Work out the finished part from the listing and answer in its coordinate system (mm). A direction names the side the tool comes from. Round coordinates to 2 decimals unless told otherwise and drop trailing zeros. Loops run counter-clockwise (first coordinate to the right, second up) from the corner with the lowest first, then second, coordinate; pieces in that order, holes last.
```python
from build123d import *

# Parameters (mm, degrees)
SCHIZZO1_W                   = 50
SCHIZZO1_H                   = 23
ESTRUSIONE_ESTRUSIONE1_DEPTH = 100
SCHIZZO2_W                   = 10
SCHIZZO2_H                   = 50
ESTRUSIONE_ESTRUSIONE2_DEPTH = 30
M7_CLEARANCE_HOLE1_D         = 7.6
ESTRUSIONE_ESTRUSIONE3_DEPTH = 60
NERVATURA2_REACH             = 125.73
SCHIZZO10_WALL_W             = 291.885494398
SCHIZZO10_WALL_H             = 5
SCHIZZO11_W                  = 30
SCHIZZO11_H                  = 30
ESTRUSIONE_ESTRUSIONE4_DEPTH = 8
TAGLIO_ESTRUSIONE1_DEPTH     = 8
RACCORDO1_R                  = 10
SMUSSO2_SIZE                 = 2
RACCORDO2_R                  = 5
SCHIZZO17_W                  = 25
SCHIZZO17_H                  = 25
ESTRUSIONE_ESTRUSIONE8_DEPTH = 3
M7_CLEARANCE_HOLE2_D         = 7.6


with BuildPart() as part:
    # Schizzo1 → Estrusione-Estrusione1 (new body)
    with BuildSketch(Plane.YZ):
        with Locations((0, 11.5)):
            Rectangle(SCHIZZO1_W, SCHIZZO1_H)
    extrude(amount=ESTRUSIONE_ESTRUSIONE1_DEPTH)

    # Schizzo2 → Estrusione-Estrusione2 (add)
    with BuildSketch(Plane.XY.offset(23)):
        with Locations((35, 0)):
            Rectangle(SCHIZZO2_W, SCHIZZO2_H)
    extrude(amount=ESTRUSIONE_ESTRUSIONE2_DEPTH)

    # M7 Clearance Hole1 (through all)
    with Locations(Plane.ZY.offset(-30)):
        with Locations((38, 0)):
            Hole(M7_CLEARANCE_HOLE1_D / 2)

    # Schizzo5 → Estrusione-Estrusione3 (add)
    with BuildSketch(Plane.YZ.offset(40)):
        Polygon((-2.124355653, 23), (2.124355653, 23), (4, 30), (-4, 30), align=None)
    extrude(amount=ESTRUSIONE_ESTRUSIONE3_DEPTH)

    # Schizzo10 wall → Nervatura2 (add, up to next)
    with BuildSketch(Plane(origin=(55, -25, 38), x_dir=(0.707106781187, 0, -0.707106781187), z_dir=(0.707106781187, 0, 0.707106781187)), mode=Mode.PRIVATE) as nervatura2_sk1:
        with Locations((0, 2.5)):
            Rectangle(SCHIZZO10_WALL_W, SCHIZZO10_WALL_H)
    nervatura2_tool1 = extrude(nervatura2_sk1.sketch, amount=-NERVATURA2_REACH, mode=Mode.PRIVATE) - part.part
    nervatura2 = nervatura2_tool1.solids().sort_by_distance((55, -25, 38))[0]
    add(nervatura2)

    # Specchia2: Nervatura2 across plane
    add(nervatura2.mirror(Plane.ZX))

    # Schizzo11 → Estrusione-Estrusione4 (add)
    with BuildSketch(Plane.YZ.offset(40)):
        with Locations((0, 38)):
            Rectangle(SCHIZZO11_W, SCHIZZO11_H)
    extrude(amount=ESTRUSIONE_ESTRUSIONE4_DEPTH)

    # Schizzo13 → Taglio-Estrusione1 (cut)
    with BuildSketch(Plane.YZ.offset(48)):
        Polygon((-6.5, 41.75277675), (-6.5, 34.24722325), (0, 30.494446501), (6.5, 34.24722325), (6.5, 41.75277675), (6.5, 53), (-6.5, 53), align=None)
    extrude(amount=-TAGLIO_ESTRUSIONE1_DEPTH, mode=Mode.SUBTRACT)

    # Schizzo16 → CSK for M3.5 Oval Head Machine Screw1 (revolve, cut)
    with BuildSketch(Plane(origin=(15, -12.5, 23), x_dir=(0, -1, 0), z_dir=(1, 0, 0))):
        Polygon((0, 0), (0, 31.171678207), (1.95, 30), (1.95, 2.15), (4.1, 0), align=None)
    csk_for_m3_5_oval_head_machine_screw1 = revolve(axis=Axis((15, -12.5, 29.35), (0, 0, -1)), mode=Mode.SUBTRACT)

    # Specchia3: CSK for M3.5 Oval Head Machine Screw1 across plane
    add(csk_for_m3_5_oval_head_machine_screw1.mirror(Plane.ZY.offset(-50)), mode=Mode.SUBTRACT)

    # Specchia3 at the second plane: CSK for M3.5 Oval Head Machine Screw1 across plane
    add(csk_for_m3_5_oval_head_machine_screw1.mirror(Plane.ZX), mode=Mode.SUBTRACT)

    # Specchia3 at the second plane copy 1 ske → Specchia3 at the second plane copy 1 (revolve, cut)
    with BuildSketch(Plane(origin=(85, 12.5, 23), x_dir=(0, 1, 0), z_dir=(-1, 0, 0))):
        Polygon((0, 0), (0, 31.171678207), (1.95, 30), (1.95, 2.15), (4.1, 0), align=None)
    revolve(axis=Axis((85, 12.5, 29.35), (0, 0, -1)), mode=Mode.SUBTRACT)

    # Raccordo1
    raccordo1_edges = [part.edges().sort_by_distance(p)[0] for p in [
        (100, 25, 11.5),
        (100, -25, 11.5),
        (0, 25, 11.5),
        (0, -25, 11.5),
    ]]
    fillet(raccordo1_edges, radius=RACCORDO1_R)

    # Smusso2
    smusso2_edges = [part.edges().sort_by_distance(p)[0] for p in [
        (44, 6.5, 53),
        (44, -6.5, 53),
    ]]
    chamfer(smusso2_edges, length=SMUSSO2_SIZE)

    # Raccordo2
    raccordo2_edges = [part.edges().sort_by_distance(p)[0] for p in [
        (30, 0, 23),
    ]]
    fillet(raccordo2_edges, radius=RACCORDO2_R)

    # Schizzo17 → Estrusione-Estrusione8 (add)
    with BuildSketch(Plane.YZ.offset(48)):
        with Locations((0, 35.5)):
            Rectangle(SCHIZZO17_W, SCHIZZO17_H)
    extrude(amount=ESTRUSIONE_ESTRUSIONE8_DEPTH)

    # M7 Clearance Hole2 (through all)
    with Locations(Plane(origin=(51, 0, 0), x_dir=(0, 0, -1), z_dir=(1, 0, 0))):
        with Locations((-38, 0)):
            Hole(M7_CLEARANCE_HOLE2_D / 2)


solid = part.part
```
1. Consider probe 1 along X at (y, z) = (-12.5, 7.75); probe 2 along Y at (x, z) = (47, 44.5); probe 3 along Y at (x, z) = (15, 15). Determine where each line is inside the solid, lowest interval first.
Answer key:
probe 1: x = 0 to 13.05, 16.95 to 83.05, 86.95 to 100
probe 2: y = -25 to -20, -15 to -6.5, 6.5 to 15, 20 to 25
probe 3: y = -25 to -14.45, -10.55 to 10.55, 14.45 to 25
2. Find section D-D (x = 49.5). Write down the section's boundary in (y, z).
Answer key:
outline: (-25, 0) - (25, 0) - (25, 43.5) - (20, 43.5) - (20, 23) - (12.5, 23) - (12.5, 48) - (-12.5, 48) - (-12.5, 23) - (-20, 23) - (-20, 43.5) - (-25, 43.5) - close; hole circle Ø7.6 at (0, 38)
3. Which of the six approach directions +Z, -Z, +X, -X, +Y, -Y give full straight-line access (tool end or side, diameter ignored) to faces 5 (the face through (44, -6.5, 43)), 6 (the face through (49, 0, 48)), 7 (the face through (49, -20, 32))?
Answer key:
face 5: +Z
face 6: +Z, +X, +Y, -Y
face 7: +Z, +X
4. Determine the mould class of faces 1 (the face through (3.01, -22.15, 11.66)), 2 (the face through (86.933, 12.246, 10.571)), 3 (the face through (83.73, -10.85, 20.98)), 4 (the face through (75, 0, 30)) for opening direction X: +X half, -X half, draft (parallel to the pull), parting line (faces both ways), or undercut.
Answer key:
face 1: -X half
face 2: undercut
face 3: undercut
face 4: draft
5. Find section C-C (z = 38). Write down the section's boundary in (x, y), then the cut area to 3 significant figures.
Answer key:
outline: (30, -25) - (55, -25) - (55, -20) - (40, -20) - (40, -15) - (48, -15) - (48, -12.5) - (51, -12.5) - (51, -3.8) - (48, -3.8) - (48, -6.5) - (40, -6.5) - (40, -3.8) - (30, -3.8) - close; (30, 3.8) - (40, 3.8) - (40, 6.5) - (48, 6.5) - (48, 3.8) - (51, 3.8) - (51, 12.5) - (48, 12.5) - (48, 15) - (40, 15) - (40, 20) - (55, 20) - (55, 25) - (30, 25) - close
area: 762 mm2
6. Find section B-B (y = -21). Write down the section's boundary in (x, z).
Answer key:
outline: (2, 0) - (98, 0) - (98, 23) - (70, 23) - (40, 53) - (30, 53) - (30, 28) arc R5 cw to (25, 23) - (2, 23) - close
7. Find section A-A (x = 15). Write down the section's boundary in (y, z), then the cut area to 3 significant figures.
Answer key:
outline: (-25, 0) - (-14.45, 0) - (-14.45, 20.85) - (-16.6, 23) - (-25, 23) - close; (-10.55, 0) - (10.55, 0) - (10.55, 20.85) - (8.4, 23) - (-8.4, 23) - (-10.55, 20.85) - close; (14.45, 0) - (25, 0) - (25, 23) - (16.6, 23) - (14.45, 20.85) - close
area: 961 mm2
8. Given pin 1 (4 mm diameter, centred on y = -2.5, z = 39, fed in from -X); pin 2 (7 mm diameter, centred on x = 68, y = 15.5, fed in from +Z); pin 3 (20 mm diameter, centred on y = 6, z = 31, fed in from +X); pin 4 (2.5 mm diameter, centred on y = -17, z = 43.5, fed in from +X), each flat-ended and moving along its own axis, determine where each tip first touches the part or whether it passes through.
Answer key:
pin 1: stops at x = 30
pin 2: stops at z = 23
pin 3: stops at x = 100
pin 4: stops at x = 40
